For this review, take the finished solid that the model builds, in its own axes (mm). Coordinates: 2 decimals unless noted, no trailing zeros. Write each loop counter-clockwise with the first axis right and the second up, starting at its lowest first coordinate (ties: lowest second). Pieces come first, ordered by that corner, then holes. Notation, with made-up numbers: M 48,-16.75 L 67,-16.75 A23 ccw 67,18.25 Z; hole C 7.25,57.5 d11. An arc over 180 degrees is marked long. One line per question, with ' | ' between items.
from build123d import *

# Parameters (mm, degrees)
ODGI_CIE_BAZOWE1_DEPTH     = 400
WYTNIJ_WYCI_GNI_CIE1_REACH = 404.597
SZKIC6_W                   = 40
SZKIC6_H                   = 20


# Sheet-metal steps are written as plain solids
with BuildPart() as part:
    # Szkic1 → Odgięcie bazowe1 (new body)
    with BuildSketch(Plane(origin=(0, 0, 0), x_dir=(1, 0, 0), z_dir=(0, 1, 0))):
        with BuildLine():
            ThreePointArc((3.992179856, 0.75), (-2.031009601, 21.810874155), (0, 0))
            Line((0, 0), (40, 0))
            Line((40, 0), (40, 0.7366))
            Line((40, 0.7366), (0, 0.7366))
            ThreePointArc((0, 0.7366), (-1.895005813, 21.08693871), (3.724848976, 1.436377273))
            Line((3.724848976, 1.436377273), (3.992179856, 0.75))
        make_face()
    extrude(amount=-ODGI_CIE_BAZOWE1_DEPTH)

    # Szkic6 → Wytnij-wyciągnięcie1 (cut, up to next)
    with BuildSketch(Plane.XY, mode=Mode.PRIVATE) as wytnij_wyci_gni_cie1_sk1:
        with Locations((20, -10)):
            Rectangle(SZKIC6_W, SZKIC6_H)
    wytnij_wyci_gni_cie1_tool1 = extrude(wytnij_wyci_gni_cie1_sk1.sketch, amount=-WYTNIJ_WYCI_GNI_CIE1_REACH, mode=Mode.PRIVATE) & part.part
    add(wytnij_wyci_gni_cie1_tool1.solids().sort_by_distance((20, -10, 0))[0], mode=Mode.SUBTRACT)


solid = part.part
1) To check wall thickness, follow line 1 along X through (y, z) = (-298, -11); line 2 along X through (y, z) = (-320.5, -10.25); line 3 along Z through (x, y) = (6.5, -179). State the ranges of each line that lie inside material, in increasing order. Write a range as [from, to].
Responses:
line 1: [-11, -10.26], [10.26, 11] | line 2: [-10.97, -10.24], [10.24, 10.97] | line 3: [-19.87, -18.94], [-3.06, -2.13], [-0.74, 0]
2) We need section A-A on z = -11. State the section outline as (x, y) points.
Responses:
outline: M -11,-400 L -10.26,-400 L -10.26,0 L -11,0 Z; M 10.26,-400 L 11,-400 L 11,0 L 10.26,0 Z
3) We need section B-B on y = -215.5. State the section outline as (x, z) points.
Responses:
outline: M 0,-0.74 L 40,-0.74 L 40,0 L 0,0 A11 ccw long 3.99,-0.75 L 3.72,-1.44 A10.26 cw long Z
4) The part is to be moulded in two halves that separate along X. For faces 1 (the cylindrical face through (-2.31, -197.2, -21)), 2 (the flat face through (9, -400, -5)), say which applies: +X half, -X half, draft (parallel to the pull), parting line (faces both ways), or undercut.
Responses:
face 1: undercut | face 2: draft
5) Insertion check: pin 1 Ø10 at (x, y) = (-3.5, -347.5) entering from +Z; pin 2 Ø4 at (x, y) = (18, -109.5) entering from -Z; pin 3 Ø0.8 at (y, z) = (-14, -0.5) entering from +X; pin 4 Ø0.8 at (x, z) = (25, -0.5) entering from +Y. Each pin has a flat end and moves straight along its axis. Give the tip position at first contact, or say it passes through.
Responses:
pin 1: z = 0 | pin 2: z = -0.74 | pin 3: x = 4.36 | pin 4: y = -20
6) We need section C-C on x = 19.5. State the section outline as (y, z) points, then the cut area to 3 significant figures.
Responses:
outline: M -400,-0.74 L -20,-0.74 L -20,0 L -400,0 Z | area: 280 mm^2
